from build123d import *

# Parameters (mm, degrees)
F0_W     = 361.95
F0_H     = 298.45
F0_R     = 4.015807
F1_DEPTH = 6.35
F0_W_2   = 368.3
F0_H_2   = 304.8
F2_DEPTH = 6.35
F3_SIZE  = 5.08


with BuildPart() as f1:
    # F0 (on Front) → F1 (new body)
    with BuildSketch(Plane.XZ):
        with Locations((-0.017055, -0.036295)):
            Rectangle(F0_W, F0_H)
        with Locations((-168.292055, -136.561295)):
            Circle(F0_R, mode=Mode.SUBTRACT)
        with Locations((168.257945, -136.561295)):
            Circle(F0_R, mode=Mode.SUBTRACT)
        with Locations((-168.292055, 136.488705)):
            Circle(F0_R, mode=Mode.SUBTRACT)
        with Locations((168.257945, 136.488705)):
            Circle(F0_R, mode=Mode.SUBTRACT)
    extrude(amount=F1_DEPTH)

    # F0 (on Front) → F2 (join)
    with BuildSketch(Plane.XZ):
        with Locations((-0.017055, -0.036295)):
            Rectangle(F0_W_2, F0_H_2)
        with Locations((-0.017055, -0.036295)):
            Rectangle(F0_W, F0_H, mode=Mode.SUBTRACT)
        with Locations((-0.017055, -0.036295)):
            Rectangle(F0_W, F0_H)
        with Locations((-168.292055, -136.561295)):
            Circle(F0_R, mode=Mode.SUBTRACT)
        with Locations((168.257945, -136.561295)):
            Circle(F0_R, mode=Mode.SUBTRACT)
        with Locations((-168.292055, 136.488705)):
            Circle(F0_R, mode=Mode.SUBTRACT)
        with Locations((168.257945, 136.488705)):
            Circle(F0_R, mode=Mode.SUBTRACT)
    extrude(amount=-F2_DEPTH)

    # F3
    f3_edges = [f1.edges().sort_by_distance(p)[0] for p in [
        (-0.017055, 6.35, 152.363705),
        (184.132945, 6.35, -0.036295),
        (-0.017055, 6.35, -152.436295),
        (-184.167055, 6.35, -0.036295),
    ]]
    chamfer(f3_edges, length=F3_SIZE)


solid = f1.part
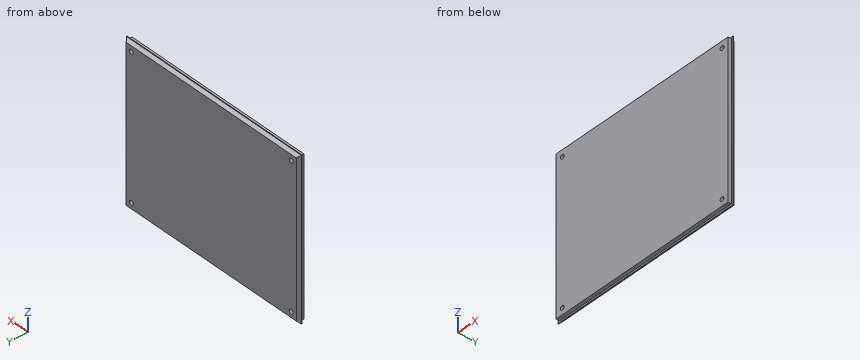
Can you work these out from the model? Positions are in its coordinate system, mm. Give positions to 0.01 mm unless a question says otherwise; leave off trailing zeros. Write each loop counter-clockwise with the first axis right and the second up, starting at its lowest first coordinate (ties: lowest second). Pieces come first, ordered by that corner, then holes. Notation, with made-up numbers: (38, 3) -> (73, 3) arc R35 cw to (73, 40) -> close; hole circle Ø5 at (89.5, 55.25). An arc over 180 degrees is marked (long way). Answer as a JSON object with one key per item and string values. Group by question number.
Item 1: Suppose I cut it at A-A (x = 92.5). Please give me the cut outline in (y, z).
Item 2: Please list where these lines run through material, in increasing order: line 1 (Z direction, x = 156, y = -5.75); line 2 (X direction, y = -2.75, z = -48.5); line 3 (Z direction, x = 56, y = 4). Write a range as [from, to].
Item 3: I'm going to push flat-ended pins straight in: P1, Ø6.5, axis at x = 168.26, z = -136.56, coming from the -Y side; P2, Ø6, axis at x = 38, y = 5, coming from the -Z side; P3, Ø3, axis at x = -61.5, y = -2.5, coming from the -Z side; P4, Ø2, axis at y = 4, z = 78, coming from the -X side. Where does each tip first touch, or does it pass through?
Item 4: Suppose I cut it at B-B (y = 4.25). Please give me the cut outline in (x, z).
Findings:
{
 "1": {"outline": "(-6.35, -149.26) -> (0, -149.26) -> (0, -152.44) -> (1.27, -152.44) -> (6.35, -147.36) -> (6.35, 147.28) -> (1.27, 152.36) -> (0, 152.36) -> (0, 149.19) -> (-6.35, 149.19) -> close"},
 "2": {"line 1": "z = [-149.26, 149.19]", "line 2": "x = [-180.99, 180.96]", "line 3": "z = [-149.71, 149.63]"},
 "3": {"P1": "passes through", "P2": "stops at z = -151.71", "P3": "stops at z = -149.26", "P4": "stops at x = -182.44"},
 "4": {"outline": "(-181.19, -149.46) -> (181.15, -149.46) -> (181.15, 149.38) -> (-181.19, 149.38) -> close; hole circle Ø8.03 at (-168.29, -136.56); hole circle Ø8.03 at (-168.29, 136.49); hole circle Ø8.03 at (168.26, -136.56); hole circle Ø8.03 at (168.26, 136.49)"}
}
